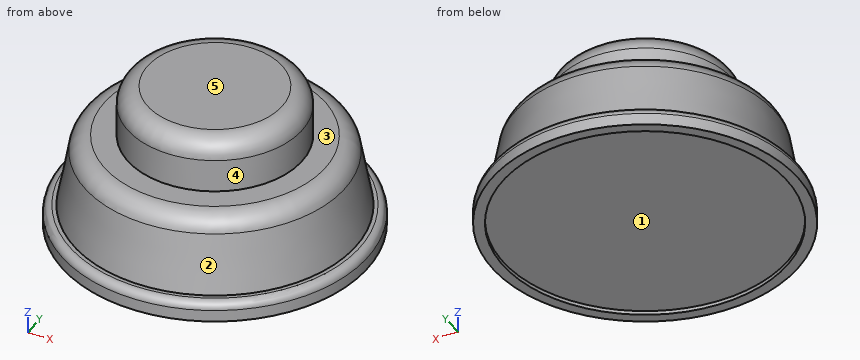
Autodesk Inventor part; units mm, degrees
ref_plane "Work Plane1" through (0, 0, 12) normal (0, 0, 1) x (1, 0, 0)
ref_plane "YZ Plane" through (0, 0, 0) normal (1, 0, 0) x (0, 1, 0)
ref_plane "XZ Plane" through (0, 0, 0) normal (0, 1, 0) x (-1, 0, 0)
sketch "Sketch1" plane through (0, 0, 0) normal (0, 0, 1) x (1, 0, 0)
  circle A0 centre (0, 0) radius 19.25
  dimension "d0" = 38.5
extrude "Extrusion1" add sketch "Sketch1" along normal blind 2.5
sketch "Sketch2" plane through (0, 0, 2.5) normal (0, 0, 1) x (1, 0, 0)
  circle A0 centre (0, 0) radius 17.75
  dimension "d3" = 35.5
ref_plane "Work Plane1" through (0, 0, 12) normal (0, 0, 1) x (1, 0, 0)
sketch "Sketch3" plane through (0, 0, 12) normal (0, 0, 1) x (1, 0, 0)
  circle A0 centre (0, 0) radius 16
  dimension "d5" = 32
loft "Loft1" add profiles "Sketch2", "Sketch3"
fillet "Fillet1" radius 2.5 1 edges at (-16, 0, 12)
fillet "Fillet2" radius 1 1 edges at (-19.25, 0, 2.5)
sketch "Sketch4" plane through (0, 0, 12) normal (0, 0, 1) x (1, 0, 0)
  circle A0 centre (0, 0) radius 11
  dimension "d12" = 22
extrude "Extrusion2" add sketch "Sketch4" along normal blind 6.7
fillet "Fillet3" radius 2.5 1 edges at (-11, 0, 18.7)
sketch "Sketch5" plane through (0, 0, 0) normal (0, 0, -1) x (-1, 0, 0)
  circle A0 centre (0, 0) radius 17.92
  circle A1 centre (0, 0) radius 19.25
  dimension "d16" = 1.33
extrude "Extrusion3" cut sketch "Sketch5" against normal blind 0.5 contours A0
properties part number "TongueSpeaker"
The listing builds one solid part. Answer for the finished solid, in the listing's coordinates (mm). Face numbers are marked on the shaded views. A direction names the side the tool comes from. Coordinates: 2 decimals unless noted, no trailing zeros. Loops run counter-clockwise (first coordinate to the right, second up) from the corner with the lowest first, then second, coordinate; pieces in that order, holes last. Notation, with made-up numbers: (68.25, 8) - (79.25, 8) arc R31 cw to (79.25, 42) - close; hole circle Ø2 at (2, -35.75). An arc over 180 degrees is marked (long way). Use a Markdown table: item, result. Add a question column.
1) The part is cut by section B-B, the plane z = 8. Give the vertices of the cut face in (x, y), and give its area (3 significant figures).
2) Find the intervals of material crossed by line 1 (Y direction, x = 0, z = 0.2); line 2 (Z direction, x = 1, y = -7); line 3 (Y direction, x = 0, z = 14.25), in increasing order.
3) The mould has two halves that part along Y. Classify the marked faces 1, 2 and 3: released by +Y, released by -Y, zero draft, split by the parting line, or undercut.
4) The part is cut by section C-C, the plane z = 3.25. Give the vertices of the cut face in (x, y).
5) Given pin 1 (5 mm diameter, centred on x = 5, z = 7, fed in from +Y); pin 2 (1.5 mm diameter, centred on x = -5, z = 15, fed in from -Y); pin 3 (4 mm diameter, centred on y = 0.5, z = 7.5, fed in from +X), each flat-ended and moving along its own axis, determine where each tip first touches the part or whether it passes through.
6) The part is cut by section A-A, the plane x = 0. Give the vertices of the cut face in (y, z).
7) For the marked faces 4 and 5, determine the directions among +Z, -Z, +X, -X, +Y, -Y from which every point of the face is accessible in a straight line to the end or side of a thin tool.
Here are the results:
| question | item | result |
|---|---|---|
| 1 | outline | circle Ø33.47 at (0, 0) |
| 1 | area | 880 mm^2 |
| 2 | line 1 | y = -19.25 to -17.92, 17.92 to 19.25 |
| 2 | line 2 | z = 0.5 to 18.7 |
| 2 | line 3 | y = -11 to 11 |
| 3 | face 1 | undercut |
| 3 | face 2 | split by the parting line |
| 3 | face 3 | zero draft |
| 4 | outline | circle Ø35.22 at (0, 0) |
| 5 | pin 1 | stops at y = 16.94 |
| 5 | pin 2 | stops at y = -10.15 |
| 5 | pin 3 | stops at x = 17.19 |
| 6 | outline | (-19.25, 0) - (-17.92, 0) - (-17.92, 0.5) - (17.92, 0.5) - (17.92, 0) - (19.25, 0) - (19.25, 1.5) arc R1 ccw to (18.25, 2.5) - (17.75, 2.5) - (16.38, 9.95) arc R2.5 ccw to (13.92, 12) - (11, 12) - (11, 16.2) arc R2.5 ccw to (8.5, 18.7) - (-8.5, 18.7) arc R2.5 ccw to (-11, 16.2) - (-11, 12) - (-13.92, 12) arc R2.5 ccw to (-16.38, 9.95) - (-17.75, 2.5) - (-18.25, 2.5) arc R1 ccw to (-19.25, 1.5) - close |
| 7 | face 4 | +Z |
| 7 | face 5 | +Z, +X, -X, +Y, -Y |
